For this review, take the finished solid that the model builds, in its own axes (mm). Face numbers are marked on the shaded views. A direction names the side the tool comes from. Give positions to 0.01 mm unless a question says otherwise; leave off trailing zeros. Order: outer loops, then holes, each group sorted by start corner. A loop starts at its lowest first (then second) coordinate and runs counter-clockwise, first axis right, second up. Notation, with made-up numbers: (-5, -39) - (0, -39) arc R9 ccw to (0, -24) - close; hole circle Ø5 at (31, -14.5). An arc over 180 degrees is marked (long way). Put each result on its own line as item: value. Start each with the question number.
```python
from build123d import *

# Parameters (mm, degrees)
SKETCH2_W           = 17.5
SKETCH2_H           = 13.5
BOSS_EXTRUDE1_DEPTH = 17.5
SKETCH4_W           = 10
SKETCH4_H           = 9.5


with BuildPart() as part:
    # Sweep1: sweep along a path in Sketch1
    with BuildLine(Plane.XY) as sweep1_path:
        Line((-26.2, 66.98), (-54.503416211, 66.98))
        ThreePointArc((-54.503416211, 66.98), (-84.493416211, 36.99), (-54.503416211, 7))
        Line((-54.503416211, 7), (203.81795526, 7))
    # Sketch2 → Sweep1 (sweep)
    with BuildSketch(Plane(origin=(203.81795526, 7, 0), x_dir=(0, 0, 1), z_dir=(-1, 0, 0))):
        with Locations((0, 6.75)):
            Rectangle(SKETCH2_W, SKETCH2_H)
    sweep(path=sweep1_path.line)

    # Sketch3 → Boss-Extrude1 (add)
    with BuildSketch(Plane.XY.offset(8.75)):
        Polygon((-26.2, 66.98), (-26.2, 53.48), (-17.2, 53.48), (-4.2, 60.98), (-4.2, 66.98), align=None)
        Polygon((203.81795526, 20.5), (203.81795526, 7), (225.81795526, 7), (225.81795526, 13), (212.81795526, 20.5), align=None)
    extrude(amount=-BOSS_EXTRUDE1_DEPTH)

    # Cut-Sweep2: sweep along a path in Sketch5
    with BuildLine(Plane.XY) as cut_sweep2_path:
        Line((-4.2, 66.98), (-26.2, 66.98))
        Line((-26.2, 66.98), (-54.503416211, 66.98))
        ThreePointArc((-54.503416211, 66.98), (-84.493416211, 36.99), (-54.503416211, 7))
        Line((-54.503416211, 7), (203.81795526, 7))
        Line((203.81795526, 7), (225.81795526, 7))
    # Sketch4 → Cut-Sweep2 (sweep, cut)
    with BuildSketch(Plane(origin=(225.81795526, 0, 0), x_dir=(0, 0, -1), z_dir=(1, 0, 0))):
        with Locations((0, 13.75)):
            Rectangle(SKETCH4_W, SKETCH4_H)
    sweep(path=cut_sweep2_path.line, mode=Mode.SUBTRACT)


solid = part.part
```
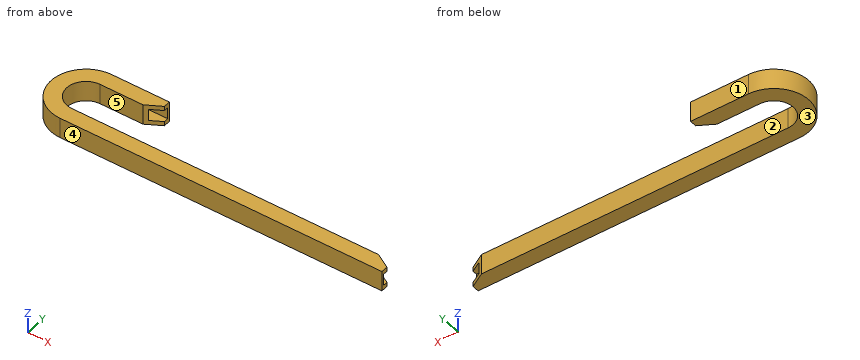
1. Add section B-B, the plane y = 36.99. Give the boundary of the cut face in (x, z), then the cut area to 3 significant figures.
2. Clearance check with flat-ended pins moving along their axes: pin 1 (1 mm diameter, centred on y = 43, z = 6.5, fed in from +X); pin 2 (8 mm diameter, centred on x = 128, z = 0, fed in from +Y); pin 3 (1 mm diameter, centred on y = 35.5, z = 3.5, fed in from -X). State where each tip first meets the part, or that it passes through.
3. The part is to be moulded in two halves that separate along Y. For the marked faces 1, 2 and 3, say which applies: released by +Y, released by -Y, zero draft, split by the parting line, or undercut.
4. Tool access review of the marked faces 4 and 5: name each direction out of +Z, -Z, +X, -X, +Y, -Y from which nothing blocks a thin tool from reaching the whole face with its end or side.
5. Wall thickness on line 1 (Y direction, x = -24, z = -4.75); line 2 (Y direction, x = 36.5, z = 1); line 3 (Z direction, x = 20.5, y = 12.5): over which ranges is each line inside the solid? List them lowest first. Write a range as from..to.
6. Add section A-A, the plane x = 112. Give the boundary of the cut face in (y, z).
Found:
1. outline: (-84.49, -8.75) - (-70.99, -8.75) - (-70.99, 8.75) - (-84.49, 8.75) - close; hole (-82.49, -5) - (-72.99, -5) - (-72.99, 5) - (-82.49, 5) - close
1. area: 141 mm^2
2. pin 1: stops at x = -69.65
2. pin 2: stops at y = 20.5
2. pin 3: stops at x = -84.48
3. face 1: released by +Y
3. face 2: undercut
3. face 3: zero draft
4. face 4: +Z, -Z, +X, -X, -Y
4. face 5: +Z, -Z, +X
5. line 1: y = 7..9, 18.5..20.5, 53.48..55.48, 64.98..66.98
5. line 2: y = 7..9, 18.5..20.5
5. line 3: z = -8.75..-5, 5..8.75
6. outline: (7, -8.75) - (20.5, -8.75) - (20.5, 8.75) - (7, 8.75) - close; hole (9, -5) - (18.5, -5) - (18.5, 5) - (9, 5) - close
